from build123d import *

# Parameters (mm, degrees)
F1_DEPTH = 15
F3_DEPTH = 2.38
F4_W     = 4
F4_H     = 4
F5_DEPTH = 18


with BuildPart() as f1:
    # F0 (on Top) → F1 (new body)
    with BuildSketch(Plane.XY):
        Polygon((-0.04099, 7.37789), (4.136275, 9.742304), (4.177265, 14.542129), (0.04099, 16.97754), (-4.136275, 14.613126), (-4.177265, 9.813301), align=None)
    extrude(amount=F1_DEPTH)

    # F2 (on face) → F3 (join)
    with BuildSketch(Plane.XY.offset(15)):
        Polygon((6.25, 15.788207), (0, 19.396646), (-6.25, 15.788207), (-6.25, 8.571329), (0, 4.96289), (6.25, 8.571329), align=None)
    extrude(amount=F3_DEPTH)

    # F4 (on face) → F5 (cut)
    with BuildSketch(Plane.XY.offset(17.38)):
        with Locations((-0.0005, 12.17989)):
            Rectangle(F4_W, F4_H)
    extrude(amount=-F5_DEPTH, mode=Mode.SUBTRACT)


solid = f1.part
The model under review builds one solid part; all positions refer to its coordinate system, in mm. A direction names the side the tool comes from. Round coordinates to 2 decimals unless told otherwise and drop trailing zeros. Write each loop counter-clockwise with the first axis right and the second up, starting at its lowest first coordinate (ties: lowest second). Pieces come first, ordered by that corner, then holes. Notation, with made-up numbers: (-18, 52) - (-14, 52) arc R11 cw to (-14, 57) - close; hole circle Ø5 at (-8, 49). An arc over 180 degrees is marked (long way). One line per item, written item: value. Start each with the question number.
1. Consider section A-A on z = 7.25. Write out the cut boundary in (x, y), and give its area (3 significant figures).
2. Clearance check with flat-ended pins moving along their axes: P1, Ø4.5, axis at x = -0.5, z = 9, coming from the -Y side; P2, Ø3, axis at y = 13.5, z = 7.5, coming from the -X side; P3, Ø4.5, axis at x = 0.5, z = 7, coming from the +Y side. State where each tip first meets the part, or that it passes through.
3. Consider section B-B on x = -1.5. Write out the cut boundary in (y, z), and give its area (3 significant figures).
4. Consider section C-C on y = 13.25. Write out the cut boundary in (x, z), and give its area (3 significant figures).
5. To check wall thickness, follow L1, parallel to Z at x = -5.25, y = 12; L2, parallel to Y at x = 1.25, z = 4.5; L3, parallel to X at y = 11, z = 9.5. State the ranges of each line that lie inside material, in increasing order. Write a range as from..to.
6. The part is to be moulded in two halves that separate along Y. For faces 1 (the face through (0, 14.18, 9)), 2 (the face through (-2.001, 12, 9)), 3 (the face through (6.25, 12, 16)), 4 (the face through (-2.02, 15.81, 7.4)), say which applies: released by +Y, released by -Y, zero draft, split by the parting line, or undercut.
7. Machinability: for faces 5 (the face through (2.14, 15.74, 7.4)), 6 (the face through (2.018, 8.544, 7.395)), 7 (the face through (-4.3, 13.9, 15)), 8 (the face through (-2.138, 8.613, 7.395)), which of the approach directions +Z, -Z, +X, -X, +Y, -Y give a long, thin tool a straight path to every point of the face, cutting with its end or side? Answer none if there is none.
8. Consider section D-D on x = 2.25. Write out the cut boundary in (y, z).
Checks:
1. outline: (-4.18, 9.81) - (-0.04, 7.38) - (4.14, 9.74) - (4.18, 14.54) - (0.04, 16.98) - (-4.14, 14.61) - close; hole (-2, 10.18) - (2, 10.18) - (2, 14.18) - (-2, 14.18) - close
1. area: 43.9 mm^2
2. P1: stops at y = 7.38
2. P2: stops at x = -4.16
2. P3: stops at y = 16.98
3. outline: (5.83, 15) - (8.24, 15) - (8.24, 0) - (10.18, 0) - (10.18, 17.38) - (5.83, 17.38) - close; (14.18, 0) - (16.11, 0) - (16.11, 15) - (18.53, 15) - (18.53, 17.38) - (14.18, 17.38) - close
3. area: 78.7 mm^2
4. outline: (-6.25, 15) - (-4.15, 15) - (-4.15, 0) - (-2, 0) - (-2, 17.38) - (-6.25, 17.38) - close; (2, 0) - (4.17, 0) - (4.17, 15) - (6.25, 15) - (6.25, 17.38) - (2, 17.38) - close
4. area: 84.9 mm^2
5. L1: z = 15..17.38
5. L2: y = 8.11..10.18, 14.18..16.27
5. L3: x = -4.17..-2, 2..4.15
6. face 1: undercut
6. face 2: undercut
6. face 3: zero draft
6. face 4: released by +Y
7. face 5: -Z, +X, +Y
7. face 6: -Z, +X, -Y
7. face 7: -Z
7. face 8: -Z, -X, -Y
8. outline: (6.26, 15) - (8.67, 15) - (8.67, 0) - (15.68, 0) - (15.68, 15) - (18.1, 15) - (18.1, 17.38) - (6.26, 17.38) - close
